For this review, take the finished solid that the model builds, in its own axes (mm). A direction names the side the tool comes from. Round coordinates to 2 decimals unless told otherwise and drop trailing zeros. Answer in a Markdown table with one row per item.
```python
from build123d import *

# Parameters (mm, degrees)
SKETCH1_W           = 8
SKETCH1_H           = 4.7625
BOSS_EXTRUDE1_DEPTH = 4.7625
CHAMFER1_SIZE       = 5.08


with BuildPart() as part:
    # Sketch1 → Boss-Extrude1 (new body)
    with BuildSketch(Plane.XY):
        Polygon((43.598645263, 118.7905), (0, 118.7905), (0, 110.6625), (5, 110.6625), (5, 105.9), (0, 105.9), (0, 72.5625), (5, 72.5625), (5, 67.8), (0, 67.8), (0, 42.8625), (5, 42.8625), (5, 38.1), (0, 38.1), (0, -38.1), (5, -38.1), (5, -42.8625), (0, -42.8625), (0, -67.8), (5, -67.8), (5, -72.5625), (0, -72.5625), (0, -105.9), (5, -105.9), (5, -110.6625), (0, -110.6625), (0, -118.7905), (43.598645263, -118.7905), (43.598645263, -110.6625), (38.598645263, -110.6625), (38.598645263, -105.9), (43.598645263, -105.9), (43.598645263, -72.5625), (38.598645263, -72.5625), (38.598645263, -67.8), (43.598645263, -67.8), (43.598645263, -42.8625), (38.598645263, -42.8625), (38.598645263, -38.1), (43.598645263, -38.1), (43.598645263, 38.1), (38.598645263, 38.1), (38.598645263, 42.8625), (43.598645263, 42.8625), (43.598645263, 67.8), (38.598645263, 67.8), (38.598645263, 72.5625), (43.598645263, 72.5625), (43.598645263, 105.9), (38.598645263, 105.9), (38.598645263, 110.6625), (43.598645263, 110.6625), align=None)
        with Locations((21.799322631, 108.28125)):
            Rectangle(SKETCH1_W, SKETCH1_H, mode=Mode.SUBTRACT)
        with Locations((21.799322631, 70.18125)):
            Rectangle(SKETCH1_W, SKETCH1_H, mode=Mode.SUBTRACT)
        with Locations((21.799322631, 40.48125)):
            Rectangle(SKETCH1_W, SKETCH1_H, mode=Mode.SUBTRACT)
        with Locations((21.799322631, -40.48125)):
            Rectangle(SKETCH1_W, SKETCH1_H, mode=Mode.SUBTRACT)
        with Locations((21.799322631, -70.18125)):
            Rectangle(SKETCH1_W, SKETCH1_H, mode=Mode.SUBTRACT)
        with Locations((21.799322631, -108.28125)):
            Rectangle(SKETCH1_W, SKETCH1_H, mode=Mode.SUBTRACT)
    extrude(amount=BOSS_EXTRUDE1_DEPTH)

    # Chamfer1
    chamfer1_edges = [part.edges().sort_by_distance(p)[0] for p in [
        (43.598645263, -118.7905, 2.38125),
        (0, -118.7905, 2.38125),
        (0, 118.7905, 2.38125),
        (43.598645263, 118.7905, 2.38125),
    ]]
    chamfer(chamfer1_edges, length=CHAMFER1_SIZE)


solid = part.part
```
Q1. Machinability: for faces 4 (the face through (41.094, 116.215, 2.348)), 5 (the face through (38.599, 108, 2)), 6 (the face through (5, 108, 2)), 7 (the face through (25.799, -41, 2)), which of the approach directions +Z, -Z, +X, -X, +Y, -Y give a long, thin tool a straight path to every point of the face, cutting with its end or side? Answer none if there is none.
Found:
| item | result |
|---|---|
| face 4 | +Z, -Z, +X, +Y |
| face 5 | +Z, -Z, +X |
| face 6 | +Z, -Z, -X |
| face 7 | +Z, -Z |
Q2. Take a section at A-A (z = 2.3). State how many separate pieces and enclosed holes the cut face has, then the cut area to 3 significant figures.
Found:
| item | result |
|---|---|
| separate pieces | 1 |
| enclosed holes | 6 |
| area | 9,790 mm² |
Q3. Insertion check: P1, Ø2.5, axis at y = 70.5, z = 2, coming from the +X side; P2, Ø2.5, axis at x = 3.5, z = 2, coming from the +Y side; P3, Ø1.4, axis at x = 1.5, z = 2, coming from the -Y side; P4, Ø2, axis at y = 36, z = 2.5, coming from the -X side. Each pin has a flat end and moves straight along its axis. Give the tip position at first contact, or say it passes through.
Found:
| item | result |
|---|---|
| P1 | x = 38.6 |
| P2 | y = 118.46 |
| P3 | y = -115.91 |
| P4 | x = 0 |
Q4. Mouldability with a two-part tool opening along X and no side actions: class faces 1 (the face through (22, -67.8, 2)), 2 (the face through (21, 2, 4.762)), 3 (the face through (5, -108, 2)) as +X half, -X half, draft (parallel to the pull), parting line (faces both ways), or undercut.
Found:
| item | result |
|---|---|
| face 1 | undercut |
| face 2 | draft |
| face 3 | -X half |
